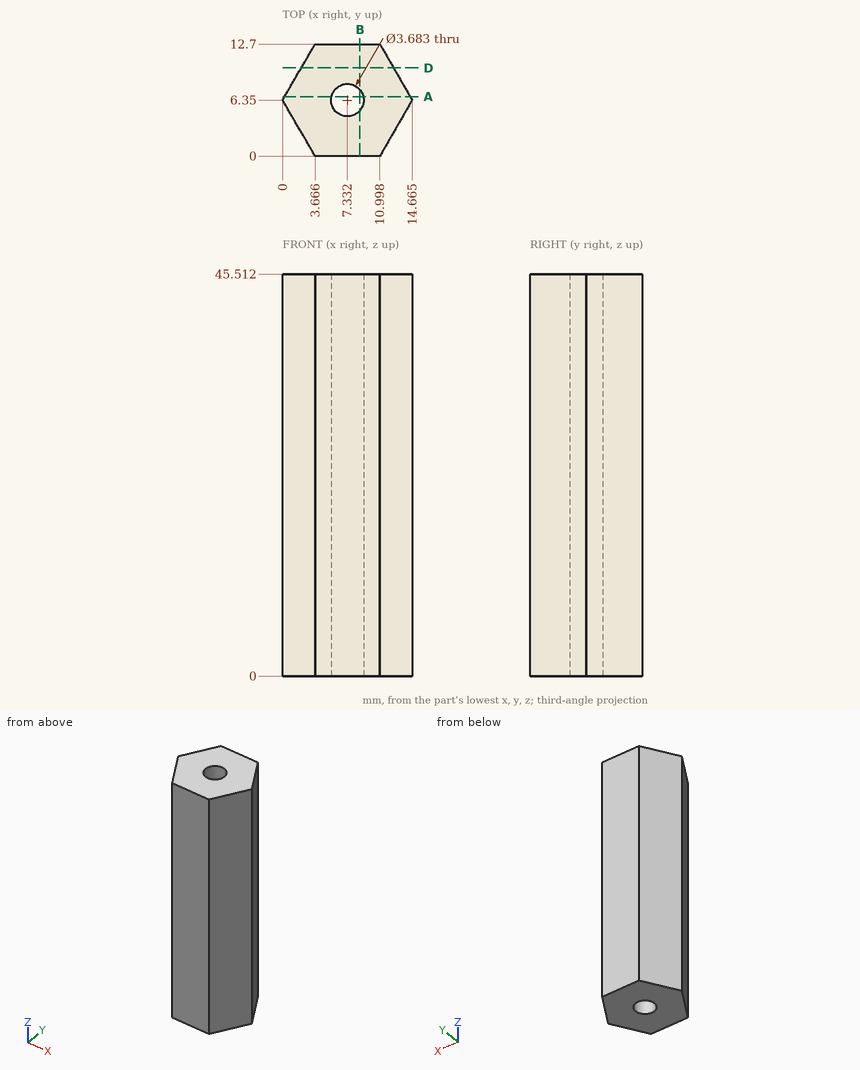
Here's the drawing with two shaded views (mm, measured from the low corner). I have some questions. Give positions to 0.01 mm unless a question says otherwise; leave off trailing zeros. Write each loop counter-clockwise with the first axis right and the second up, starting at its lowest first coordinate (ties: lowest second). Pieces come first, ordered by that corner, then holes. Notation, with made-up numbers: (42.5, 5) -> (70.5, 5) arc R31 cw to (70.5, 44) -> close; hole circle Ø4 at (71, 82.25). An arc over 180 degrees is marked (long way). One line per item, written item: value.
Q1. Imagine slicing it at D-D on y = 10. Please give me the cut outline in (x, z).
Results found:
outline: (2.11, 0) -> (12.56, 0) -> (12.56, 45.51) -> (2.11, 45.51) -> close
Q2. Please list where these lines run through material, in increasing order: line 1 (Y direction, x = 6, z = 9); line 2 (Y direction, x = 6.5, z = 19); line 3 (X direction, y = 7.5, z = 36) (1 decimal). Write a range as [from, to].
Results found:
line 1: y = [0, 5.08], [7.62, 12.7]
line 2: y = [0, 4.71], [7.99, 12.7]
line 3: x = [0.7, 5.9], [8.8, 14]
Q3. Imagine slicing it at A-A on y = 6.75. Please give me the cut outline in (x, z) (1 decimal).
Results found:
outline: (0.2, 0) -> (5.5, 0) -> (5.5, 45.5) -> (0.2, 45.5) -> close; (9.1, 0) -> (14.4, 0) -> (14.4, 45.5) -> (9.1, 45.5) -> close
Q4. For P1, Ø1, axis at x = 12, z = 30.5, coming from the +Y side; P2, Ø4, axis at y = 4, z = 32, coming from the -X side; P3, Ø4, axis at y = 10.5, z = 10.5, coming from the +X side, each with a flat end and sliding along its axis, tell me the tip position at first contact or that it passes through.
Results found:
P1: stops at y = 11.83
P2: stops at x = 0.2
P3: stops at x = 13.42
Q5. Imagine slicing it at B-B on x = 8.75. Please give me the cut outline in (y, z) (1 decimal), and give its area (3 significant figures).
Results found:
outline: (0, 0) -> (5.2, 0) -> (5.2, 45.5) -> (0, 45.5) -> close; (7.5, 0) -> (12.7, 0) -> (12.7, 45.5) -> (7.5, 45.5) -> close
area: 471 mm^2
